The listing builds one solid part. Answer for the finished solid, in the listing's coordinates (mm). Face numbers are marked on the shaded views. A direction names the side the tool comes from. Give positions to 0.01 mm unless a question says otherwise; leave off trailing zeros. Write each loop counter-clockwise with the first axis right and the second up, starting at its lowest first coordinate (ties: lowest second). Pieces come first, ordered by that corner, then holes. Notation, with made-up numbers: (52, 56.5) - (83, 56.5) arc R25 ccw to (83, 79.5) - close; hole circle Ø5 at (-26.5, 19). An arc over 180 degrees is marked (long way). Answer as CSV lines item,"result". Start each with the question number.
(1) For the marked faces 5 and 6, determine the directions among +Z, -Z, +X, -X, +Y, -Y from which every point of the face is accessible in a straight line to the end or side of a thin tool.
(2) Find section D-D (x = 2.75). Write down the section's boundary in (y, z).
(3) Straight lines are drawn through the part: probe 1 along Z at (x, y) = (-1.75, 3.5); probe 2 along Z at (x, y) = (-7.75, 8); probe 3 along X at (y, z) = (6.25, 4.5). For each, find the intervals that lie inside material, in ascending order.
(4) Find section B-B (y = -1.75). Write down the section's boundary in (x, z), then the cut area to 3 significant figures.
(5) For a pull along Z with two mould halves and no side action, classify the marked faces 1, 2, 3 and 4 as pulls with the +Z half, pulls with the -Z half, needs draft (parallel to the pull), parting line crosses it, or undercut.
(6) Each of these flat-tipped pins is pushed along its axis until it touches: pin 1 Ø5 at (y, z) = (-6.5, 46) entering from +X; pin 2 Ø1.5 at (y, z) = (0, 40) entering from -X; pin 3 Ø6 at (x, z) = (-2, 53) entering from -Y; pin 4 Ø2 at (x, y) = (2, 1) entering from +Z. Where does it stop, or does it pass through?
(7) Find section C-C (z = 11). Write down the section's boundary in (x, y), then the cut area to 3 significant figures.
(8) Find section A-A (x = 0). Write down the section's boundary in (y, z), then the cut area to 3 significant figures.
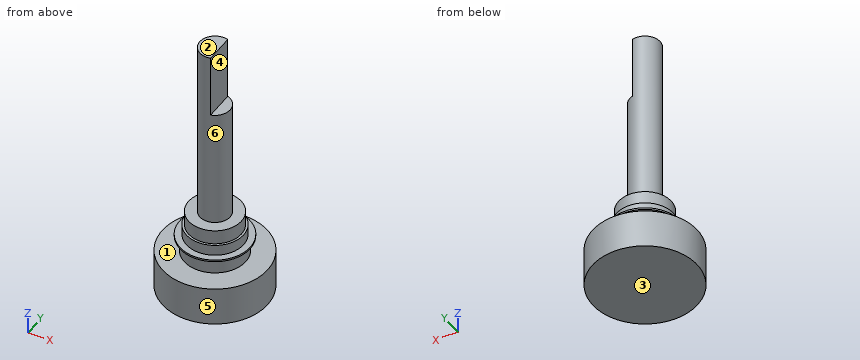
from build123d import *

# Parameters (mm, degrees)
SKETCH2_R           = 11.95
BOSS_EXTRUDE1_DEPTH = 8.9
SKETCH3_R           = 7
BOSS_EXTRUDE2_DEPTH = 3.7
SKETCH5_R           = 8
BOSS_EXTRUDE3_DEPTH = 0.4
SKETCH6_R           = 6.5
BOSS_EXTRUDE4_DEPTH = 2.5
SKETCH7_R           = 6
BOSS_EXTRUDE5_DEPTH = 3.3
SKETCH8_R           = 3.45
BOSS_EXTRUDE6_DEPTH = 41.8
CUT_EXTRUDE2_START  = -14.49
CUT_EXTRUDE2_DEPTH  = 14.49


with BuildPart() as part:
    # Sketch2 → Boss-Extrude1 (new body)
    with BuildSketch(Plane(origin=(0, 0, 0), x_dir=(0, 1, 0), z_dir=(0, 0, 1))):
        with Locations(Location((0, 0, 0), (0, 0, 270))):
            Circle(SKETCH2_R)
    extrude(amount=BOSS_EXTRUDE1_DEPTH)

    # Sketch3 → Boss-Extrude2 (add)
    with BuildSketch(Plane.XY.offset(8.9)):
        Circle(SKETCH3_R)
    extrude(amount=BOSS_EXTRUDE2_DEPTH)

    # Sketch5 → Boss-Extrude3 (add)
    with BuildSketch(Plane.XY.offset(12.6)):
        Circle(SKETCH5_R)
    extrude(amount=BOSS_EXTRUDE3_DEPTH)

    # Sketch6 → Boss-Extrude4 (add)
    with BuildSketch(Plane.XY.offset(13)):
        Circle(SKETCH6_R)
    extrude(amount=BOSS_EXTRUDE4_DEPTH)

    # Sketch7 → Boss-Extrude5 (add)
    with BuildSketch(Plane.XY.offset(15.5)):
        Circle(SKETCH7_R)
    extrude(amount=BOSS_EXTRUDE5_DEPTH)

    # Sketch8 → Boss-Extrude6 (add)
    with BuildSketch(Plane.XY.offset(18.8)):
        Circle(SKETCH8_R)
    extrude(amount=BOSS_EXTRUDE6_DEPTH)

    # Sketch10 → Cut-Extrude2 (cut)
    with BuildSketch(Plane.XY.offset(60.6).offset(CUT_EXTRUDE2_START)):
        with BuildLine():
            Line((0.95, 3.31662479), (0.95, -3.31662479))
            ThreePointArc((0.95, -3.31662479), (3.45, 0), (0.95, 3.31662479))
        make_face()
    extrude(amount=CUT_EXTRUDE2_DEPTH, mode=Mode.SUBTRACT)


solid = part.part
Result set:
1,face 5,"+Z, -Z"
1,face 6,"+Z"
2,outline,"(-11.63, 0) - (11.63, 0) - (11.63, 8.9) - (6.44, 8.9) - (6.44, 12.6) - (7.51, 12.6) - (7.51, 13) - (5.89, 13) - (5.89, 15.5) - (5.33, 15.5) - (5.33, 18.8) - (2.08, 18.8) - (2.08, 46.11) - (-2.08, 46.11) - (-2.08, 18.8) - (-5.33, 18.8) - (-5.33, 15.5) - (-5.89, 15.5) - (-5.89, 13) - (-7.51, 13) - (-7.51, 12.6) - (-6.44, 12.6) - (-6.44, 8.9) - (-11.63, 8.9) - close"
3,probe 1,"0 to 18.8"
3,probe 2,"0 to 8.9"
3,probe 3,"-10.19 to 10.19"
4,outline,"(-11.82, 0) - (11.82, 0) - (11.82, 8.9) - (6.78, 8.9) - (6.78, 12.6) - (7.81, 12.6) - (7.81, 13) - (6.26, 13) - (6.26, 15.5) - (5.74, 15.5) - (5.74, 18.8) - (2.97, 18.8) - (2.97, 46.11) - (0.95, 46.11) - (0.95, 60.6) - (-2.97, 60.6) - (-2.97, 18.8) - (-5.74, 18.8) - (-5.74, 15.5) - (-6.26, 15.5) - (-6.26, 13) - (-7.81, 13) - (-7.81, 12.6) - (-6.78, 12.6) - (-6.78, 8.9) - (-11.82, 8.9) - close"
4,area,"555 mm^2"
5,face 1,"undercut"
5,face 2,"pulls with the +Z half"
5,face 3,"pulls with the -Z half"
5,face 4,"needs draft"
6,pin 1,"through"
6,pin 2,"x = -3.45"
6,pin 3,"y = -3.45"
6,pin 4,"z = 46.11"
7,outline,"circle Ø14 at (0, 0)"
7,area,"154 mm^2"
8,outline,"(-11.95, 0) - (11.95, 0) - (11.95, 8.9) - (7, 8.9) - (7, 12.6) - (8, 12.6) - (8, 13) - (6.5, 13) - (6.5, 15.5) - (6, 15.5) - (6, 18.8) - (3.45, 18.8) - (3.45, 60.6) - (-3.45, 60.6) - (-3.45, 18.8) - (-6, 18.8) - (-6, 15.5) - (-6.5, 15.5) - (-6.5, 13) - (-8, 13) - (-8, 12.6) - (-7, 12.6) - (-7, 8.9) - (-11.95, 8.9) - close"
8,area,"631 mm^2"
